Could you check a few things on this model? Use its own coordinates, in mm. Round coordinates to 2 decimals unless told otherwise and drop trailing zeros. Loops run counter-clockwise (first coordinate to the right, second up) from the corner with the lowest first, then second, coordinate; pieces in that order, holes last. Notation, with made-up numbers: (18, 73) -> (70, 73) arc R21 ccw to (70, 89) -> close; hole circle Ø10 at (75.25, 61). An arc over 180 degrees is marked (long way). Write each question's results on one line, items separated by ' | '.
from build123d import *

# Parameters (mm, degrees)
SKETCH_1_R          = 33
EXTRUDE_1_DEPTH     = 16
SKETCH_2_R          = 4.1
SKETCH_2_R_2        = 1.45
CUT_EXTRUDE_1_DEPTH = 16


with BuildPart() as part:
    # 草图1 → 凸台-拉伸1 (new body)
    with BuildSketch(Plane(origin=(0, 0, 0), x_dir=(0, 0, -1), z_dir=(1, 0, 0))):
        Circle(SKETCH_1_R)
    extrude(amount=EXTRUDE_1_DEPTH)

    # 草图2 → 切除-拉伸1 (cut)
    with BuildSketch(Plane.ZY):
        Circle(SKETCH_2_R)
        with Locations((-7.071067812, 7.071067812)):
            Circle(SKETCH_2_R_2)
        with Locations((-7.071067812, -7.071067812)):
            Circle(SKETCH_2_R_2)
        with Locations((7.071067812, -7.071067812)):
            Circle(SKETCH_2_R_2)
        with Locations((7.071067812, 7.071067812)):
            Circle(SKETCH_2_R_2)
    extrude(amount=-CUT_EXTRUDE_1_DEPTH, mode=Mode.SUBTRACT)


solid = part.part
1) I want a section at A-A, the plane z = 0. Write out the boundary of the cut face in (x, y).
Model answer:
outline: (0, -33) -> (16, -33) -> (16, -4.1) -> (0, -4.1) -> close; (0, 4.1) -> (16, 4.1) -> (16, 33) -> (0, 33) -> close
2) I'm going to push flat-ended pins straight in: pin 1 (4 mm diameter, centred on x = 3, y = -9, fed in from -Z); pin 2 (2.5 mm diameter, centred on y = 7.07, z = 7.07, fed in from -X); pin 3 (1.5 mm diameter, centred on x = 13.5, z = -8, fed in from -Y); pin 4 (1 mm diameter, centred on x = 3.5, y = 7, fed in from +Z). Where does each tip first touch, or does it pass through?
Model answer:
pin 1: stops at z = -32.25 | pin 2: passes through | pin 3: stops at y = -32.19 | pin 4: stops at z = 32.35
3) I want a section at C-C, the plane x = 5. Write out the boundary of the cut face in (y, z), plus the area to 3 significant figures.
Model answer:
outline: circle Ø66 at (0, 0); hole circle Ø2.9 at (-7.07, -7.07); hole circle Ø2.9 at (-7.07, 7.07); hole circle Ø8.2 at (0, 0); hole circle Ø2.9 at (7.07, -7.07); hole circle Ø2.9 at (7.07, 7.07) | area: 3,340 mm2
4) If we mould it in two halves opening along Z, with no side actions, what happens to faces 1 (the cylindrical face through (7.9, -12.6, -30.5)), 2 (the cylindrical face through (7.888, 6.516, 8.41)), 3 (the flat face through (16, -7, 0))? For each: released by +Z, released by -Z, zero draft, split by the parting line, or undercut.
Model answer:
face 1: split by the parting line | face 2: undercut | face 3: zero draft
5) I want a section at D-D, the plane z = 22. Write out the boundary of the cut face in (x, y), plus the area to 3 significant figures.
Model answer:
outline: (0, -24.6) -> (16, -24.6) -> (16, 24.6) -> (0, 24.6) -> close | area: 787 mm2
6) I need wall thicknesses on line 1 (Y direction, x = 9.25, z = 0); line 2 (Y direction, x = 11, z = -4.5); line 3 (Z direction, x = 5.5, y = 20). Which ranges of each line are inside material? Lowest first, please.
Model answer:
line 1: y = -33 to -4.1, 4.1 to 33 | line 2: y = -32.69 to 32.69 | line 3: z = -26.25 to 26.25
